Model file for the job. Use its own axes, mm. A direction names the side the tool comes from. Give positions to 0.01 mm unless a question says otherwise; leave off trailing zeros. Order: outer loops, then holes, each group sorted by start corner. A loop starts at its lowest first (then second) coordinate and runs counter-clockwise, first axis right, second up. Notation, with made-up numbers: (-25.75, 15.5) - (6.25, 15.5) arc R27 ccw to (6.25, 52.5) - close; hole circle Ø7 at (51, 0.5). An arc over 180 degrees is marked (long way). Use CSV: the item, a comma, the result in double quotes. Start each with the question number.
(1) Tool access for faces 1 (the cylindrical face through (-74.223, 43.93, 280.035)), 2 (the flat face through (-32.9, 45, 297)), 3 (the flat face through (-82.021, 44.042, 277.723)), 4 (the flat face through (-73.106, 44, 270)), 5 (the flat face through (35.9, 45, 297)): list every direction of +Z, -Z, +X, -X, +Y, -Y with a clear straight run to the whole face (end or side of a thin tool).
(2) Pull direction Z, two halves, no side cores. Call faces 6 (the cylindrical face through (-56.2, 45.8, 275.4)), 7 (the flat face through (-7, 41, 244)), 8 (the flat face through (2, 44, 287.61)): +Z half, -Z half, draft (parallel to the pull), parting line (faces both ways), or undercut.
(3) Band-saw the part on B-B, the plane x = -42.5. Give the cut face in (y, z), then the cut area to 3 significant figures.
(4) Band-saw the part on D-D, the plane x = -64. Give the cut face in (y, z).
(5) Band-saw the part on A-A, the plane z = 295.61. Give the cut face in (x, y).
(6) Probe L1, parallel to X at y = 43.25, z = 295.61; L2, parallel to Z at x = -8, y = 42.5; L3, parallel to Z at x = 17.5, y = 41.75. List the from-to ranges inside material, lowest first.
(7) Drop flat-ended pins along their axis: pin 1 Ø4 at (x, y) = (-75.82, 44) entering from -Z; pin 2 Ø1.8 at (x, y) = (-74.5, 44) entering from +Z; pin 3 Ø4 at (y, z) = (44, 294) entering from -X. Give the stop position or say it passes through.
(8) Band-saw the part on C-C, the plane z = 222.5. Give the cut face in (x, y).
from build123d import *

# Parameters (mm, degrees)
SKETCH119_R     = 4.25
PAD037_DEPTH    = 8
POCKET089_DEPTH = 10
SKETCH145_W     = 212.757988
SKETCH145_H     = 111.377136
POCKET090_DEPTH = 2
CHAMFER024_SIZE = 7.9
SKETCH146_W     = 16
SKETCH146_H     = 8
SKETCH146_W_2   = 8
SKETCH146_H_2   = 16
PAD043_DEPTH    = 6
POCKET091_DEPTH = 6
SKETCH148_R     = 5.25
POCKET092_DEPTH = 2
CHAMFER025_SIZE = 0.5
SKETCH149_W     = 7.25
SKETCH149_H     = 2.4
POCKET093_DEPTH = 6
SKETCH150_R     = 1.6
POCKET094_DEPTH = 11.42
SKETCH151_R     = 1.6
POCKET095_DEPTH = 10.75


with BuildPart() as part:
    # Sketch119 → Pad037 (new body)
    with BuildSketch(Plane.XZ):
        with BuildLine():
            Line((43.1, 311.61), (58.9, 311.61))
            Line((58.9, 311.61), (58.9, 287.61))
            Line((58.9, 287.61), (68.0627698178, 182.8790617439))
            ThreePointArc((-62.6189518066, 287.61), (-20.1922299081, 206.652605958), (68.0627698178, 182.8790617439))
            Line((-9.9, 287.61), (-62.6189518066, 287.61))
            Line((-9.9, 311.61), (-9.9, 287.61))
            Line((5.9, 311.61), (-9.9, 311.61))
            Line((5.9, 287.61), (5.9, 311.61))
            Line((43.1, 287.61), (5.9, 287.61))
            Line((43.1, 287.61), (43.1, 311.61))
        make_face()
        with Locations((51.1, 295.61)):
            Circle(SKETCH119_R, mode=Mode.SUBTRACT)
    extrude(amount=PAD037_DEPTH)

    # Sketch144 (on Sketch) → Pocket089 (cut, symmetric)
    with BuildSketch(Plane(origin=(0, -2, 0), x_dir=(1, 0, 0), z_dir=(0, 1, 0))):
        with BuildLine():
            Line((46.4683764269, -270.2884951656), (51.3899439591, -195.7125763223))
            ThreePointArc((51.3899439591, -195.7125763223), (22.163397434, -200.2401058051), (-4.4606389833, -213.1183910114))
            Line((43.6500461, -271.0604538296), (-4.4606389833, -213.1183910114))
            Line((46.4683764269, -270.2884951656), (43.6500461, -271.0604538296))
        make_face()
        with BuildLine():
            Line((38.2664280008, -273.5828375694), (-45.585449, -273.501129))
            ThreePointArc((-12.4277002687, -219.1620599694), (-33.4458091568, -243.6227695917), (-45.585449, -273.501129))
            Line((40.8654991159, -272.1768310477), (-12.4277002687, -219.1620599694))
            Line((38.2664280008, -273.5828375694), (40.8654991159, -272.1768310477))
        make_face()
    extrude(amount=POCKET089_DEPTH, both=True, mode=Mode.SUBTRACT)

    # Sketch145 (on Face4 of Pocket089) → Pocket090 (cut)
    with BuildSketch(Plane(origin=(0, 0, 0), x_dir=(1, 0, 0), z_dir=(0, 1, 0))):
        with Locations((0.739727, -231.921432)):
            Rectangle(SKETCH145_W, SKETCH145_H)
    extrude(amount=-POCKET090_DEPTH, mode=Mode.SUBTRACT)

    # Chamfer024
    chamfer024_edges = [part.edges().sort_by_distance(p)[0] for p in [
        (51, 0, 311.61),
        (-2, 0, 311.61),
    ]]
    chamfer(chamfer024_edges, length=CHAMFER024_SIZE)

    # Sketch146 (on Face24 of Chamfer024) → Pad043 (join)
    with BuildSketch(Plane(origin=(0, -2, 0), x_dir=(1, 0, 0), z_dir=(0, 1, 0))):
        with Locations((-69.7716084762, -283.61)):
            Rectangle(SKETCH146_W, SKETCH146_H)
        with Locations((64.0627698178, -174.8790617439)):
            Rectangle(SKETCH146_W_2, SKETCH146_H_2)
    extrude(amount=-PAD043_DEPTH)

    # Sketch147 (on Face26 of Pad043) → Pocket091 (cut)
    with BuildSketch(Plane(origin=(0, -2, 0), x_dir=(1, 0, 0), z_dir=(0, 1, 0))):
        Polygon((59.8525224324, -181.7142315678), (60.0816034962, -186.6062288871), (55.6003748066, -190.8009391349), (45.9859602644, -189.8230627729), (46.188335, -187.833328), (54.8977345384, -188.7191558264), (58.040592409, -185.7772443485), (57.8465339537, -181.633150432), align=None)
        Polygon((-62.4277412024, -277.4774293102), (-56.5131742791, -277.9036519615), (-52.105898537, -274.2887258472), (-52.105898537, -264.8339163664), (-50.105898537, -264.8339163664), (-50.105898537, -275.234992563), (-55.8614558604, -279.9558032607), (-62.5714948328, -279.4722563437), align=None)
    extrude(amount=-POCKET091_DEPTH, mode=Mode.SUBTRACT)

    # Sketch148 (on Face42 of Pocket091) → Pocket092 (cut)
    with BuildSketch(Plane(origin=(0, -2, 0), x_dir=(1, 0, 0), z_dir=(0, 1, 0))):
        with Locations((-32.5660026534, -280.61)):
            Circle(SKETCH148_R)
        with Locations((58.1, -210.8987256618)):
            Circle(SKETCH148_R)
    extrude(amount=-POCKET092_DEPTH, mode=Mode.SUBTRACT)

    # Chamfer025
    chamfer025_edges = [part.edges().sort_by_distance(p)[0] for p in [
        (52.85, -2, 210.898726),
        (-37.816003, -2, 280.61),
    ]]
    chamfer(chamfer025_edges, length=CHAMFER025_SIZE)

    # Sketch149 (on Face1 of Chamfer025) → Pocket093 (cut)
    with BuildSketch(Plane(origin=(0, -2, 0), x_dir=(1, 0, 0), z_dir=(0, 1, 0))):
        with Locations((-52.8400088116, -283.61)):
            Rectangle(SKETCH149_W, SKETCH149_H)
        Polygon((62.6335907882, -185.2715531365), (62.0017116533, -192.4939646977), (64.3925789287, -192.7031384803), (65.0244580636, -185.4807269191), align=None)
    extrude(amount=-POCKET093_DEPTH, mode=Mode.SUBTRACT)

    # Sketch150 (on Face6 of Pocket093) → Pocket094 (cut)
    with BuildSketch(Plane(origin=(0, 0, 287.61), x_dir=(-1, 0, 0), z_dir=(0, 0, 1))):
        with Locations((52.8216084762, 5)):
            Circle(SKETCH150_R)
    extrude(amount=-POCKET094_DEPTH, mode=Mode.SUBTRACT)

    # Sketch151 (on Face5 of Pocket094) → Pocket095 (cut)
    with BuildSketch(Plane(origin=(83.4240645156, 0, 7.2986599104), x_dir=(-0.0871557427, 0, 0.9961946981), z_dir=(0.9961946981, 0, 0.0871557427))):
        with Locations((182.7510904443, 5)):
            Circle(SKETCH151_R)
    extrude(amount=-POCKET095_DEPTH, mode=Mode.SUBTRACT)


with BuildPart() as part_1:
    # Body028 placement: moved
    add(part.part.moved(Location((-23, 49, 0))))


solid = part_1.part
Answer block:
1,face 1,"+Z"
1,face 2,"+Z, -X, +Y, -Y"
1,face 3,"-X, +Y, -Y"
1,face 4,"+Y, -Y"
1,face 5,"+Z, +X, +Y, -Y"
2,face 6,"undercut"
2,face 7,"draft"
2,face 8,"+Z half"
3,outline,"(41, 206.1) - (47, 206.1) - (47, 225.71) - (41, 225.71) - close; (41, 273.53) - (47, 273.53) - (47, 287.61) - (41, 287.61) - close"
3,area,"202 mm2"
4,outline,"(41, 228.43) - (47, 228.43) - (47, 258.75) - (41, 258.75) - close; (41, 273.51) - (47, 273.51) - (47, 287.61) - (41, 287.61) - close"
5,outline,"(-32.9, 41) - (-17.1, 41) - (-17.1, 49) - (-32.9, 49) - close; (20.1, 41) - (23.85, 41) - (23.85, 49) - (20.1, 49) - close; (32.35, 41) - (35.9, 41) - (35.9, 49) - (32.35, 49) - close"
6,L1,"x = -32.9 to -17.1, 20.1 to 23.85, 32.35 to 35.9"
6,L2,"z = 187.48 to 202.77, 236.56 to 246.45, 273.56 to 287.61"
6,L3,"z = 182.1 to 196.37, 267.27 to 271.81, 272.37 to 287.61"
7,pin 1,"stops at z = 244.54"
7,pin 2,"stops at z = 287.61"
7,pin 3,"stops at x = -32.9"
8,outline,"(-59.37, 41) - (-39.2, 41) - (-39.2, 47) - (-59.37, 47) - close; (-32.07, 41) - (-19.67, 41) - (-19.67, 47) - (-32.07, 47) - close; (26.62, 41) - (41.6, 41) - (41.6, 47) - (26.62, 47) - close"
